The model under review builds one solid part; all positions refer to its coordinate system, in mm. A direction names the side the tool comes from. Coordinates: 2 decimals unless noted, no trailing zeros. Order: outer loops, then holes, each group sorted by start corner. A loop starts at its lowest first (then second) coordinate and runs counter-clockwise, first axis right, second up. Notation, with made-up numbers: M -19,44.5 L 4,44.5 A20 ccw 4,56.5 Z; hole C 86.25,-20 d2. An arc over 180 degrees is marked long. One line per item, written item: value.
```python
from build123d import *

# Parameters (mm, degrees)
F1_DEPTH = 19.05


with BuildPart() as f1:
    # F0 (on Front) → F1 (new body)
    with BuildSketch(Plane.XZ):
        with BuildLine():
            Line((-142.719461, 108.376235), (-142.719461, -132.923765))
            Line((-142.719461, -132.923765), (-117.319461, -132.923765))
            Line((-117.319461, -132.923765), (-117.319461, -142.448765))
            Line((-117.319461, -142.448765), (-66.519461, -142.448765))
            Line((-66.519461, -142.448765), (-66.519461, -132.923765))
            Line((-66.519461, -132.923765), (85.880539, -132.923765))
            Line((85.880539, -132.923765), (85.880539, -142.448765))
            Line((85.880539, -142.448765), (136.680539, -142.448765))
            Line((136.680539, -142.448765), (136.680539, -132.923765))
            Line((136.680539, -132.923765), (162.080539, -132.923765))
            Line((162.080539, -132.923765), (162.080539, 336.976235))
            ThreePointArc((162.080539, 336.976235), (150.921307, 363.917003), (123.980539, 375.076235))
            ThreePointArc((123.980539, 375.076235), (-64.60484, 296.961613), (-142.719461, 108.376235))
        make_face()
    extrude(amount=F1_DEPTH)


solid = f1.part
```
(1) Insertion check: pin 1 Ø7.5 at (y, z) = (-5, -138.5) entering from +X; pin 2 Ø7.5 at (y, z) = (-5.5, -137.5) entering from -X; pin 3 Ø3 at (x, y) = (-22, -15.5) entering from +Z. Each pin has a flat end and moves straight along its axis. Give the tip position at first contact, or say it passes through.
Geometry results:
pin 1: stops at x = 136.68
pin 2: stops at x = -117.32
pin 3: stops at z = 332.55
(2) For L1, parallel to X at y = -3.75, z = 141.5; L2, parallel to Z at x = 111.5, y = -18; L3, parallel to X at y = -10.5, z = 196, list the stretches that pass through material, from the lowest coordinate up.
Geometry results:
L1: x = -140.65 to 162.08
L2: z = -142.45 to 374.78
L3: x = -127.91 to 162.08
(3) We need section B-B, the plane z = 297. State the section outline as (x, y) points.
Geometry results:
outline: M -64.57,-19.05 L 162.08,-19.05 L 162.08,0 L -64.57,0 Z
(4) We need section A-A, the plane y = -12.75. State the section outline as (x, z) points.
Geometry results:
outline: M -142.72,-132.92 L -117.32,-132.92 L -117.32,-142.45 L -66.52,-142.45 L -66.52,-132.92 L 85.88,-132.92 L 85.88,-142.45 L 136.68,-142.45 L 136.68,-132.92 L 162.08,-132.92 L 162.08,336.98 A38.1 ccw 123.98,375.08 A266.7 ccw -142.72,108.38 Z
(5) Mouldability with a two-part tool opening along X and no side actions: class faces 4 (the flat face through (85.881, -9, -138)), 5 (the flat face through (111, -9, -142.449)), 6 (the flat face through (162.081, -9, 99)) as +X half, -X half, draft (parallel to the pull), parting line (faces both ways), or undercut.
Geometry results:
face 4: undercut
face 5: draft
face 6: +X half
(6) Tool access review of faces 1 (the flat face through (136.681, -9, -138)), 2 (the flat face through (-117.319, -9, -138)), 3 (the flat face through (9, -9, -132.924)): name each direction out of +Z, -Z, +X, -X, +Y, -Y from which nothing blocks a thin tool from reaching the whole face with its end or side.
Geometry results:
face 1: -Z, +X, +Y, -Y
face 2: -Z, -X, +Y, -Y
face 3: -Z, +Y, -Y
(7) We need section C-C, the plane x = -44. State the section outline as (y, z) points, plus the area to 3 significant figures.
Geometry results:
outline: M -19.05,-132.92 L 0,-132.92 L 0,315.53 L -19.05,315.53 Z
area: 8,540 mm2
